from build123d import *

# Parameters (mm, degrees)
SKETCH1_R           = 3.98
BOSS_EXTRUDE1_DEPTH = 6
CHAMFER1_SIZE       = 1.5


with BuildPart() as part:
    # Sketch1 → Boss-Extrude1 (new body)
    with BuildSketch(Plane(origin=(0, 0, 0), x_dir=(1, 0, 0), z_dir=(0, 1, 0))):
        with BuildLine():
            Line((-5.521270529, 3.430097921), (-20.521270529, 3.430097921))
            ThreePointArc((-20.521270529, 3.430097921), (-32.542541057, 0), (-20.521270529, -3.430097921))
            Line((-20.521270529, -3.430097921), (-5.521270529, -3.430097921))
            ThreePointArc((-5.521270529, -3.430097921), (6.5, 0), (-5.521270529, 3.430097921))
        make_face()
        with Locations(Location((-26.042541057, 0, 0), (0, 0, 270))):
            Circle(SKETCH1_R, mode=Mode.SUBTRACT)
        with Locations(Location((0, 0, 0), (0, 0, 270))):
            Circle(SKETCH1_R, mode=Mode.SUBTRACT)
    extrude(amount=BOSS_EXTRUDE1_DEPTH)

    # Chamfer1
    chamfer1_edges = [part.edges().sort_by_distance(p)[0] for p in [
        (-32.542541057, 0, 0),
        (-32.542541057, 6, 0),
        (6.5, 6, 0),
        (6.5, 0, 0),
    ]]
    chamfer(chamfer1_edges, length=CHAMFER1_SIZE)


solid = part.part
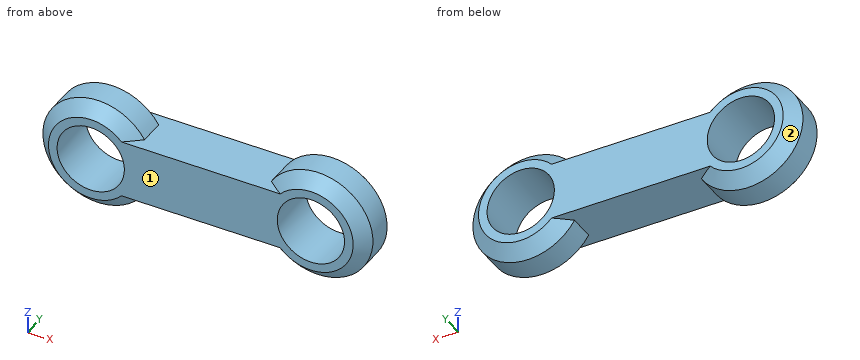
Check sheet for the modelled part. Datum: model origin and axes. Units: mm. Face numbers are marked on the shaded views. Round coordinates to 2 decimals unless told otherwise and drop trailing zeros. Order: outer loops, then holes, each group sorted by start corner. A loop starts at its lowest first (then second) coordinate and runs counter-clockwise, first axis right, second up.
(1) Draft check along X on the marked faces 1 and 2. Enter one of: pulls with the +X half, pulls with the -X half, needs draft (parallel to the pull), parting line crosses it, or undercut.
(2) Scan lines: probe 1 along X at (y, z) = (3.35, 0); probe 2 along X at (y, z) = (2, -2.75); probe 3 along Z at (x, y) = (-10, 1.25). Record each from-to range of solid material in increasing order.
(3) Go/stop test with flat-tipped pins: P1, Ø7, axis at x = -26.04, z = 0, coming from the +Y side (3 decimals); P2, Ø3, axis at x = -11.5, y = 4, coming from the +Z side; P3, Ø1.5, axis at x = -17.5, y = 3, coming from the -Z side; P4, Ø1.5, axis at x = -17, z = 3.5, coming from the -Y side. Record where each tip stops, or that it passes through.
(4) Cross-section at A-A, the plane z = 0. Enter the section's corners in (x, y), and give its area (3 significant figures).
(5) Cross-section at B-B, the plane x = 0. Enter the section's corners in (y, z), and give its area (3 significant figures).
(6) Cross-section at D-D, the plane x = -19. Enter the section's corners in (y, z).
(7) Cross-section at C-C, the plane y = 2. Enter the section's corners in (x, z).
Check sheet entries:
1. face 1: needs draft
1. face 2: undercut
2. probe 1: x = -32.54 to -30.02, -22.06 to -3.98, 3.98 to 6.5
2. probe 2: x = -31.93 to -28.92, -23.17 to -2.88, 2.88 to 5.89
2. probe 3: z = -3.43 to 3.43
3. P1: passes through
3. P2: stops at z = 3.43
3. P3: stops at z = -3.43
3. P4: stops at y = 0
4. outline: (-32.54, 1.5) - (-31.04, 0) - (-30.02, 0) - (-30.02, 6) - (-31.04, 6) - (-32.54, 4.5) - close; (-22.06, 0) - (-3.98, 0) - (-3.98, 6) - (-22.06, 6) - close; (3.98, 0) - (5, 0) - (6.5, 1.5) - (6.5, 4.5) - (5, 6) - (3.98, 6) - close
4. area: 134 mm2
5. outline: (0, -5) - (1.5, -6.5) - (4.5, -6.5) - (6, -5) - (6, -3.98) - (0, -3.98) - close; (0, 3.98) - (6, 3.98) - (6, 5) - (4.5, 6.5) - (1.5, 6.5) - (0, 5) - close
5. area: 25.7 mm2
6. outline: (0, -3.43) - (6, -3.43) - (6, 3.43) - (0, 3.43) - close
7. outline: (-20.52, -3.43) - (-5.52, -3.43) arc R6.5 ccw (long way) to (-5.52, 3.43) - (-20.52, 3.43) arc R6.5 ccw (long way) to start; hole circle Ø7.96 at (-26.04, 0); hole circle Ø7.96 at (0, 0)
